Could you check a few things on this model? Use its own coordinates, in mm. Face numbers are marked on the shaded views. A direction names the side the tool comes from. Give positions to 0.01 mm unless a question says otherwise; leave off trailing zeros. Loops run counter-clockwise (first coordinate to the right, second up) from the corner with the lowest first, then second, coordinate; pieces in that order, holes last. Notation, with made-up numbers: (79, -14) - (131, -14) arc R20 ccw to (131, 3) - close; hole circle Ø9 at (-32, -36). An arc over 180 degrees is marked (long way). Answer in a Markdown table with one row per item. Add a question column.
```python
from build123d import *

# Parameters (mm, degrees)
F0_W        = 99.0999639034
F0_H        = 102.6097461581
F1_DEPTH    = 50.8
F2_R        = 25.1416200386
F3_T1_DEPTH = 227.8741153204
F4_R        = 7.4465956944
F4_R_2      = 7.6481080303
F5_DEPTH    = 155.448
F6_W        = 76.1274546385
F6_H        = 70.1917465776
F7_DEPTH    = 112.268
F8_T1_DEPTH = 76.1274546385


# Not quite as in the source:
# - a fillet or chamfer that OpenCascade refuses, or shapes differently, is made with other operations: its cross-section is extruded or revolved along the edge and cut away or added


with BuildPart() as f1:
    # F0 (on Front) → F1 (new body)
    with BuildSketch(Plane.XZ):
        Rectangle(F0_W, F0_H)
    extrude(amount=F1_DEPTH)

    # F2
    f2_edges = [f1.edges().sort_by_distance(p)[0] for p in [
        (0, -50.8, 51.304873),
        (0, 0, 51.304873),
    ]]
    fillet(f2_edges, radius=F2_R)

    # F3: fillet of radius 25.7548302834 on 2 edges, made by hand

    # F3_s2 → F3_t1 (cut)
    with BuildSketch(Plane.YZ.offset(-113.9370576602)):
        with BuildLine():
            ThreePointArc((0, -25.5500427957), (-7.5434151417, -43.7614579374), (-25.7548302834, -51.3048730791))
            Line((-25.7548302834, -51.3048730791), (0, -51.3048730791))
            Line((0, -51.3048730791), (0, -25.5500427957))
        make_face()
        with BuildLine():
            ThreePointArc((-50.8, -25.5500427957), (-43.2565848583, -43.7614579374), (-25.0451697166, -51.3048730791))
            Line((-25.0451697166, -51.3048730791), (-50.8, -51.3048730791))
            Line((-50.8, -51.3048730791), (-50.8, -25.5500427957))
        make_face()
    extrude(amount=F3_T1_DEPTH, mode=Mode.SUBTRACT)

    # F4 (on face) → F5 (cut)
    with BuildSketch(Plane(origin=(-49.5499819517, 0, 0), x_dir=(0, -1, 0), z_dir=(-1, 0, 0))):
        with Locations((25.1416200386, 26.1632530405)):
            Circle(F4_R)
        with Locations((25.7548302834, -25.5500427957)):
            Circle(F4_R_2)
    extrude(amount=-F5_DEPTH, mode=Mode.SUBTRACT)

    # F6 (on Front) → F7 (cut)
    with BuildSketch(Plane.XZ):
        with Locations((1.9891783595, 22.4027493969)):
            Rectangle(F6_W, F6_H)
    extrude(amount=F7_DEPTH, mode=Mode.SUBTRACT)

    # F8: fillet of radius 25.1416200386 on 2 edges, made by hand

    # F8_s2 → F8_t1 (cut)
    with BuildSketch(Plane.YZ.offset(-36.0745489597)):
        with BuildLine():
            ThreePointArc((-50.8, -37.8347439305), (-43.4361899807, -20.0569339112), (-25.6583799614, -12.6931238919))
            Line((-25.6583799614, -12.6931238919), (-50.8, -12.6931238919))
            Line((-50.8, -12.6931238919), (-50.8, -37.8347439305))
        make_face()
        with BuildLine():
            ThreePointArc((0, -37.8347439305), (-7.3638100193, -20.0569339112), (-25.1416200386, -12.6931238919))
            Line((-25.1416200386, -12.6931238919), (0, -12.6931238919))
            Line((0, -12.6931238919), (0, -37.8347439305))
        make_face()
    extrude(amount=F8_T1_DEPTH, mode=Mode.SUBTRACT)


solid = f1.part
```
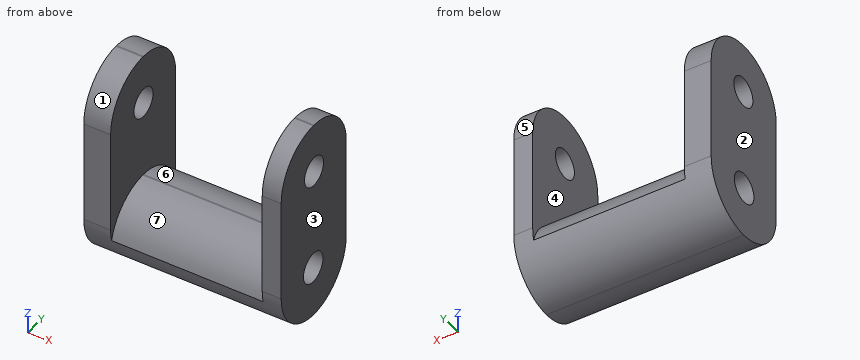
(1) I want a section at B-B on x = 28. Please give me the cut outline in (y, z).
(2) We'd pull the mould along X, two halves only. Please class the marked faces 1, 2, 3 and 4: pulls with the +X half, pulls with the -X half, needs draft (parallel to the pull), parting line crosses it, or undercut.
(3) I want a section at D-D on y = -44. Please give me the cut outline in (x, z).
(4) On a 3-axis mill with a long thin cutter (end or side, diameter ignored), from which of +Z, -Z, +X, -X, +Y, -Y can I reach the whole of each face in a straight line? I mean the marked faces 5, 6 and 7. Say none if no direction works.
(5) For pin 1 Ø5 at (x, y) = (26, -8.5) entering from +Z; pin 2 Ø2 at (x, y) = (37, -18) entering from +Z; pin 3 Ø13.5 at (y, z) = (-25.14, 26.16) entering from -X; pin 4 Ø2 at (x, y) = (-34.5, -28.5) entering from +Z, each with a flat end and sliding along its axis, tell me the tip position at first contact or that it passes through.
(6) Please list where these lines run through material, in increasing order: line 1 (X direction, y = -13.5, z = 10); line 2 (Z direction, x = -41.5, y = -29); line 3 (Z direction, x = 16.5, y = -22.5).
(7) I want a section at A-A on z = 1. Please give me the cut outline in (x, y), then the cut area to 3 significant figures.
(8) I want a section at C-C on y = -29. Please give me the cut outline in (x, z).
Reported:
| question | item | result |
|---|---|---|
| 1 | outline | (-50.05, -31.73) arc R25.75 ccw to (-25.4, -51.3) arc R25.75 ccw to (-0.75, -31.73) arc R25.14 ccw to (-25.14, -12.69) - (-25.66, -12.69) arc R25.14 ccw to start; hole circle Ø15.3 at (-25.75, -25.55) |
| 2 | face 1 | needs draft |
| 2 | face 2 | pulls with the -X half |
| 2 | face 3 | pulls with the +X half |
| 2 | face 4 | undercut |
| 3 | outline | (-49.55, -42.99) - (49.55, -42.99) - (49.55, 43.36) - (40.05, 43.36) - (40.05, -20.64) - (-36.07, -20.64) - (-36.07, 43.36) - (-49.55, 43.36) - close |
| 4 | face 5 | +Z, +X, -X, +Y |
| 4 | face 6 | +Z, +Y |
| 4 | face 7 | +Z, -Y |
| 5 | pin 1 | z = -17.05 |
| 5 | pin 2 | z = -13.45 |
| 5 | pin 3 | through |
| 5 | pin 4 | z = -12.76 |
| 6 | line 1 | -49.55 to -36.07, 40.05 to 49.55 |
| 6 | line 2 | -51 to -32.48, -18.62 to 19.79, 32.53 to 51.08 |
| 6 | line 3 | -51.1 to -32.47, -18.63 to -12.83 |
| 7 | outline | (-49.55, -50.8) - (-36.07, -50.8) - (-36.07, 0) - (-49.55, 0) - close; (40.05, -50.8) - (49.55, -50.8) - (49.55, 0) - (40.05, 0) - close |
| 7 | area | 1,170 mm² |
| 8 | outline | (-49.55, -51) - (49.55, -51) - (49.55, -32.48) - (-49.55, -32.48) - close; (-49.55, -18.62) - (49.55, -18.62) - (49.55, 19.79) - (40.05, 19.79) - (40.05, -12.92) - (-36.07, -12.92) - (-36.07, 19.79) - (-49.55, 19.79) - close; (-49.55, 32.53) - (-36.07, 32.53) - (-36.07, 51.08) - (-49.55, 51.08) - close; (40.05, 32.53) - (49.55, 32.53) - (49.55, 51.08) - (40.05, 51.08) - close |
